Autodesk Inventor part; units mm, degrees
ref_plane "Work Plane1" through (0, 0, 0) normal (0, -1, 0) x (1, 0, 0)
ref_plane "YZ Plane" through (0, 0, 0) normal (1, 0, 0) x (0, 1, 0)
ref_plane "XZ Plane" through (0, 0, 0) normal (0, 1, 0) x (-1, 0, 0)
sketch "Sketch1" plane through (0, 0, 0) normal (1, 0, 0) x (0, 1, 0)
  circle A0 centre (0, 0) radius 7.45
  circle A1 centre (0, 0) radius 4.1
  dimension "d0" = 8.2
  dimension "d1" = 14.9
extrude "Body" add sketch "Sketch1" along normal blind 2.1
sketch "Sketch2" plane through (0, 0, 0) normal (0, 0, 1) x (1, 0, 0)
  line L0 (0, -4.1) -> (0, 4.1)
  line L1 (2.1, 7.45) -> (2.1, -7.45)
  line L2 (-1.2, 0) -> (7.2, 0)
  line L3 (0, -0.42) -> (2.1, 0.3443)
  line L4 (0, 0.42) -> (2.1, 1.1843)
  dimension "d4" = 0.42
  dimension "d5" = 0.42
  dimension "d6" = 70
extrude "Cut" cut sketch "Sketch2" along normal up to next contours L0 L2 L3 | L0 L4 L1 L3 L2
ref_plane "Work Plane1" through (0, 0, 0) normal (0, -1, 0) x (1, 0, 0)
equation "\"d0\" = SD1"
equation "\"d1\" = SD2"
equation "\"d2\" = SD"
equation "\"d4\" = 0.2 * SD"
equation "\"d5\" = 0.2 * SD"
equation "\"d6\" = FAWI"
equation "\"d7\" = SD"
equation "\"SD1\" = 8.2"
equation "\"SD2\" = 14.9"
equation "\"SD\" = 2.1"
equation "\"FAWI\" = 70deg"
equation "\"NND\" = 8"
properties part number "AS 1968 - 1976 - 8" material "Steel, Mild"
CAD build for the part. Positions are in the model's coordinates, mm. A direction names the side the tool comes from. Give positions to 0.01 mm unless a question says otherwise; leave off trailing zeros. Write each loop counter-clockwise with the first axis right and the second up, starting at its lowest first coordinate (ties: lowest second). Pieces come first, ordered by that corner, then holes. Notation, with made-up numbers: (-3.75, -7.75) -> (38.25, -7.75) arc R7 cw to (38.25, 0.25) -> close; hole circle Ø4 at (67, -3.75). An arc over 180 degrees is marked (long way). Write each question's results on one line, items separated by ' | '.
1. Wall check: probe 1 along Y at (x, z) = (0.95, 0); probe 2 along Z at (x, y) = (0.55, 0); probe 3 along Y at (x, z) = (1.6, -2.5). Give the ranges that are in metal, low to high. Write a range as [from, to].
Geometry check:
probe 1: [-7.45, -4.1], [4.1, 7.45] | probe 2: [-7.45, -4.1] | probe 3: [-7.02, -3.25], [3.25, 7.02]
2. Two-plate mould, pull along Y, no slides. Class faces 3 (the flat face through (1.04, 0.8, 5.66)), 4 (the flat face through (0, 3.2, -3.2)): pulls with the +Y half, pulls with the -Y half, needs draft (parallel to the pull), parting line crosses it, or undercut.
Geometry check:
face 3: undercut | face 4: needs draft
3. Cut at D-D, the plane y = 6.25. Write the cut outline in (x, z).
Geometry check:
outline: (0, -4.05) -> (2.1, -4.05) -> (2.1, 4.05) -> (0, 4.05) -> close
4. Cut at C-C, the plane x = 0.4. Write the cut outline in (y, z), then the cut area to 3 significant figures.
Geometry check:
outline: (-0.27, 4.09) -> (-0.27, 7.44) arc R7.45 ccw (long way) to (0.57, 7.43) -> (0.57, 4.06) arc R4.1 cw (long way) to start | area: 119 mm²
5. Cut at A-A, the plane z = 2.25. Write the cut outline in (x, y).
Geometry check:
outline: (0, -7.1) -> (2.1, -7.1) -> (2.1, -3.43) -> (0, -3.43) -> close; (0, 3.43) -> (2.1, 3.43) -> (2.1, 7.1) -> (0, 7.1) -> close
6. Which spindle directions (+Z, -Z, +X, -X, +Y, -Y) get a long thin tool onto all of the face, cutting with end or side? Do faces 1 (the flat face through (2.1, 3.2, -3.2)), 2 (the flat face through (1.04, -0.04, 5.74)). Say none if no direction does.
Geometry check:
face 1: +Z, -Z, +X, +Y, -Y | face 2: +Z, -X
7. Cut at B-B, the plane y = -1. Write the cut outline in (x, z).
Geometry check:
outline: (0, -7.38) -> (2.1, -7.38) -> (2.1, -3.98) -> (0, -3.98) -> close; (0, 3.98) -> (2.1, 3.98) -> (2.1, 7.38) -> (0, 7.38) -> close
8. Drop flat-ended pins along their axis: P1, Ø1, axis at x = 1.5, y = 2.5, coming from the +Z side; P2, Ø1, axis at x = 0.5, z = -3, coming from the +Y side. Give the stop position or say it passes through.
Geometry check:
P1: z = 7.18 | P2: y = 7.02
